Verification items for the finished model (mm, model axes). A direction names the side the tool comes from. Coordinates: 2 decimals unless noted, no trailing zeros. Loops run counter-clockwise (first coordinate to the right, second up) from the corner with the lowest first, then second, coordinate; pieces in that order, holes last. Notation, with made-up numbers: (65.25, 63) -> (117.25, 63) arc R8 ccw to (117.25, 70) -> close; hole circle Ø5 at (82, 84). An arc over 180 degrees is marked (long way). Write item = value, one per line.
```python
from build123d import *

# Parameters (mm, degrees)
BOSS_EXTRUDE1_START = -317.5
SKETCH4_R           = 2.54
SKETCH4_R_2         = 9.525
SKETCH4_R_3         = 14.2875
BOSS_EXTRUDE1_DEPTH = 3.175
BOSS_EXTRUDE2_DEPTH = 3.175
BOSS_EXTRUDE3_START = -76.2
BOSS_EXTRUDE3_DEPTH = 3.175
SKETCH9_R           = 2.54
CUT_EXTRUDE2_DEPTH  = 506.024067921
LPATTERN1_COUNT     = 10
LPATTERN1_PITCH     = 50.8
SKETCH13_W          = 25.4
SKETCH13_H          = 139.7
CUT_EXTRUDE4_DEPTH  = 506.024067921


with BuildPart() as part:
    # Sketch4 → Boss-Extrude1 (new body)
    with BuildSketch(Plane(origin=(0, 0, 0), x_dir=(0, 0, -1), z_dir=(1, 0, 0)).offset(BOSS_EXTRUDE1_START)):
        with BuildLine():
            Line((362.853219884, 88.9), (0, 88.9))
            Line((0, 88.9), (0, 65.0875))
            ThreePointArc((0, 65.0875), (14.2875, 50.8), (0, 36.5125))
            Line((0, 36.5125), (0, 12.7))
            Line((0, 12.7), (362.853219884, 12.7))
            Line((362.853219884, 12.7), (362.853219884, 88.9))
        make_face()
        with Locations((53.34, 25.4)):
            Circle(SKETCH4_R, mode=Mode.SUBTRACT)
        with Locations((53.34, 50.8)):
            Circle(SKETCH4_R_2, mode=Mode.SUBTRACT)
        with Locations((177.45964, 50.8)):
            Circle(SKETCH4_R_3, mode=Mode.SUBTRACT)
        with Locations((53.34, 76.2)):
            Circle(SKETCH4_R, mode=Mode.SUBTRACT)
        with Locations((337.453219884, 53.975)):
            Circle(SKETCH4_R_3, mode=Mode.SUBTRACT)
    extrude(amount=-BOSS_EXTRUDE1_DEPTH)

    # Sketch7 → Boss-Extrude2 (add)
    with BuildSketch(Plane(origin=(0, 88.9, 0), x_dir=(1, 0, 0), z_dir=(0, 1, 0))):
        Polygon((-319.0875, 0), (-342.9, 0), (-342.9, 362.853219884), (-317.5, 362.853219884), align=None)
    extrude(amount=-BOSS_EXTRUDE2_DEPTH)

    # Sketch7<2> → Boss-Extrude3 (add)
    with BuildSketch(Plane(origin=(0, 88.9, 0), x_dir=(1, 0, 0), z_dir=(0, 1, 0)).offset(BOSS_EXTRUDE3_START)):
        Polygon((-319.0875, 0), (-342.9, 0), (-342.9, 362.853219884), (-317.5, 362.853219884), align=None)
    extrude(amount=BOSS_EXTRUDE3_DEPTH)

    # Sketch9 → Cut-Extrude2 (cut, through all)
    with BuildSketch(Plane(origin=(0, 88.9, 0), x_dir=(1, 0, 0), z_dir=(0, 1, 0))):
        with Locations(Location((-330.2, 355.6, 0), (0, 0, 270))):
            Circle(SKETCH9_R)
    cut_extrude2 = extrude(amount=-CUT_EXTRUDE2_DEPTH, mode=Mode.SUBTRACT)

    # LPattern1: Cut-Extrude2 ×10
    with Locations(*[(0, 0, i * LPATTERN1_PITCH) for i in range(1, LPATTERN1_COUNT)]):
        add(cut_extrude2, mode=Mode.SUBTRACT)

    # Mirror1: part across face


with BuildPart() as part_1:
    add(part.part)
    add(part.part.mirror(Plane(origin=(-320.239664948, 22.265914948, 0), x_dir=(1, 0, 0), z_dir=(0, 0, 1))))

    # Sketch13 → Cut-Extrude4 (cut, through all)
    with BuildSketch(Plane(origin=(0, 88.9, 0), x_dir=(1, 0, 0), z_dir=(0, 1, 0))):
        with Locations((-330.2, 293.003219884)):
            Rectangle(SKETCH13_W, SKETCH13_H)
        with Locations((-330.2, -293.003219884)):
            Rectangle(SKETCH13_W, SKETCH13_H)
    extrude(amount=-CUT_EXTRUDE4_DEPTH, mode=Mode.SUBTRACT)


solid = part_1.part
```
1) Release check for a two-part mould opening along Z. For faces 3 (the face through (-319.065, 53.661, -62.425)), 4 (the face through (-330, 12.7, -3)), 5 (the face through (-320, 51, 223.153)) record: pulls with the +Z half, pulls with the -Z half, needs draft (parallel to the pull), parting line crosses it, or undercut.
Ans:
face_3 = undercut
face_4 = needs draft
face_5 = pulls with the +Z half
2) Sectioned sample at A-A, the plane x = -338.75. Record the cut outline in (y, z) (3 decimals).
Ans:
outline = (12.7, -223.153) -> (15.875, -223.153) -> (15.875, 223.153) -> (12.7, 223.153) -> close; (85.725, -223.153) -> (88.9, -223.153) -> (88.9, 223.153) -> (85.725, 223.153) -> close
3) Sectioned sample at D-D, the plane z = -39.5. Record the cut outline in (x, y) (3 decimals).
Ans:
outline = (-342.9, 12.7) -> (-317.5, 12.7) -> (-317.5, 88.9) -> (-342.9, 88.9) -> (-342.9, 85.725) -> (-320.675, 85.725) -> (-320.675, 15.875) -> (-342.9, 15.875) -> close
4) Sectioned sample at C-C, the plane z = -170. Record the cut outline in (x, y) (1 decimal), plus the area to 3 significant figures.
Ans:
outline = (-342.9, 12.7) -> (-317.5, 12.7) -> (-317.5, 38.6) -> (-320.7, 38.6) -> (-320.7, 15.9) -> (-342.9, 15.9) -> close; (-342.9, 85.7) -> (-320.7, 85.7) -> (-320.7, 63) -> (-317.5, 63) -> (-317.5, 88.9) -> (-342.9, 88.9) -> close
area = 306 mm2
5) Tool access check on faces 1 (the face through (-319.065, 51.428, 163.186)), 2 (the face through (-332, 85.725, 3)). Record the directions out of +Z, -Z, +X, -X, +Y, -Y that give a thin tool (end or side, any length) a straight path to the whole face; none if there is none.
Ans:
face_1 = +X, -X
face_2 = +Z, -Z, -X
6) Sectioned sample at B-B, the plane y = 50.8. Record the cut outline in (x, z) (1 decimal).
Ans:
outline = (-320.7, -223.2) -> (-317.5, -223.2) -> (-317.5, -191.7) -> (-320.7, -191.7) -> close; (-320.7, -163.2) -> (-317.5, -163.2) -> (-317.5, -62.9) -> (-320.7, -62.9) -> close; (-320.7, -43.8) -> (-317.5, -43.8) -> (-317.5, -14.3) -> (-320.7, -14.3) -> close; (-320.7, 14.3) -> (-317.5, 14.3) -> (-317.5, 43.8) -> (-320.7, 43.8) -> close; (-320.7, 62.9) -> (-317.5, 62.9) -> (-317.5, 163.2) -> (-320.7, 163.2) -> close; (-320.7, 191.7) -> (-317.5, 191.7) -> (-317.5, 223.2) -> (-320.7, 223.2) -> close
7) Depth check by flat-ended pin: pin 1 Ø1.5 at (y, z) = (80, -120.5) entering from -X (3 decimals). Enter the tip coordinate at first touch or a pass-through.
Ans:
pin_1 = -320.675
8) Material ranges on line 1 (Y direction, x = -333.75, z = -130.5) (3 decimals); line 2 (X direction, y = 87.7, z = -152.4); line 3 (Z direction, x = -318.5, y = 40.5), recorded low to high.
Ans:
line_1 = 12.7 to 15.875, 85.725 to 88.9
line_2 = -342.9 to -332.74, -327.66 to -317.5
line_3 = -223.15 to -187.36, -167.56 to -9.9, 9.9 to 167.56, 187.36 to 223.15
